Build history of the part. All positions in model axes, mm. Give positions to 0.01 mm unless a question says otherwise; leave off trailing zeros. Loops run counter-clockwise (first coordinate to the right, second up) from the corner with the lowest first, then second, coordinate; pieces in that order, holes last. Notation, with made-up numbers: M 79.25,12 L 113.25,12 A7 ccw 113.25,21 Z; hole C 46,86.25 d1. An arc over 180 degrees is marked long. Answer as a JSON object with one key per item and string values. Group by question number.
1. Drop flat-ended pins along their axis: pin 1 Ø2.5 at (x, y) = (-10.61, 259.5) entering from +Z; pin 2 Ø4.5 at (x, y) = (19.14, 230.6) entering from +Z. Give the stop position or say it passes through.
2. Slice it at B-B (z = 54.9). Give the number of separate pieces and of enclosed holes in the cut face, then the cut area to 3 significant figures.
3. Drill centre lines: line 1 along X through (y, z) = (248, 54.05); line 2 along X through (y, z) = (259, 55.2); line 3 along X through (y, z) = (231, 55.5). Where is each one in solid material? Low to high. Write a range as [from, to].
4. Slice it at C-C (x = -13). List the corners of the cut face in (y, z).
5. Slice it at A-A (x = 9). List the corners of the cut face in (y, z).
6. Mould opens along X. For faces 1 (the face through (34.622, 229.133, 54.721)), 2 (the face through (-28, 226.353, 55)), 3 (the face through (-41.107, 257, 55)) say: released by +X, released by -X, zero draft, split by the parting line, or undercut.
from build123d import *

# Parameters (mm, degrees)
SKETCH_1_R                                   = 3
SKETCH_1_R_2                                 = 4.5
EXTRUDE_1_DEPTH                              = 3
CSK_FOR_M3_HEX_SOCKET_COUNTERSUNK_HE_2_COUNT = 2
CSK_FOR_M3_HEX_SOCKET_COUNTERSUNK_HE_2_PITCH = 42.898135158
SKETCH_2_R                                   = 1.5
SKETCH_2_R_2                                 = 1.25
CUT_EXTRUDE1_DEPTH                           = 10
SKETCH4_R                                    = 1.25
CUT_EXTRUDE2_DEPTH                           = 3


with BuildPart() as part:
    # Эскиз1 → Бобышка-Вытянуть1 (new body)
    with BuildSketch(Plane.XY.offset(53.2)):
        with BuildLine():
            Line((-4.102180416, 226.353254388), (38.893407272, 226.353254388))
            Line((38.893407272, 226.353254388), (38.893407272, 286.353254388))
            Line((38.893407272, 286.353254388), (-41.106592728, 286.353254388))
            Line((-41.106592728, 286.353254388), (-41.106592728, 226.353254388))
            Line((-41.106592728, 226.353254388), (-15.28891158, 226.353254388))
            ThreePointArc((-15.28891158, 226.353254388), (-9.695545998, 229.144425829), (-4.102180416, 226.353254388))
        make_face()
        with Locations((0.393407272, 249.403254388)):
            Circle(SKETCH_1_R, mode=Mode.SUBTRACT)
        with Locations((14.393407272, 249.403254388)):
            Circle(SKETCH_1_R, mode=Mode.SUBTRACT)
        with Locations((-29.150473778, 261.95614373)):
            Circle(SKETCH_1_R_2, mode=Mode.SUBTRACT)
        with Locations((10.923063266, 261.985726175)):
            Circle(SKETCH_1_R_2, mode=Mode.SUBTRACT)
    extrude(amount=EXTRUDE_1_DEPTH)

    # Sketch3 → CSK for M3 Hex Socket Countersunk Head Screw1 (revolve, cut)
    with BuildSketch(Plane(origin=(3.643407272, 270.603254388, 56.2), x_dir=(0, -1, 0), z_dir=(1, 0, 0))):
        Polygon((0, 0), (0, 3), (1.7, 3), (1.7, 1.77), (3.47, 0), align=None)
    csk_for_m3_hex_socket_countersunk_head_s = revolve(axis=Axis((3.643407272, 270.603254388, 62.55), (0, 0, -1)), mode=Mode.SUBTRACT)

    # CSK for M3 Hex Socket Countersunk He 2: CSK for M3 Hex Socket Countersunk Head Screw1 ×2
    with Locations(*[Vector(0.36132106775864725, -0.9324414651836066, 0) * (i * CSK_FOR_M3_HEX_SOCKET_COUNTERSUNK_HE_2_PITCH) for i in range(1, CSK_FOR_M3_HEX_SOCKET_COUNTERSUNK_HE_2_COUNT)]):
        add(csk_for_m3_hex_socket_countersunk_head_s, mode=Mode.SUBTRACT)

    # Эскиз2 → Cut-Extrude1 (cut)
    with BuildSketch(Plane.XY.offset(56.2)):
        with Locations((-28.106592728, 240.603254388)):
            Circle(SKETCH_2_R)
        with Locations((-10.606592728, 259.503254388)):
            Circle(SKETCH_2_R)
        with Locations((3.643407272, 270.603254388)):
            Circle(SKETCH_2_R_2)
        with Locations((19.143407272, 230.603254388)):
            Circle(SKETCH_2_R_2)
    extrude(amount=-CUT_EXTRUDE1_DEPTH, mode=Mode.SUBTRACT)

    # Sketch4 → Cut-Extrude2 (cut)
    with BuildSketch(Plane.XY.offset(56.2)):
        with Locations((-9.606592728, 276.603254388)):
            Circle(SKETCH4_R)
        with Locations((-19.620743586, 239.653254388)):
            Circle(SKETCH4_R)
        with Locations((34.893407272, 230.353254388)):
            Circle(SKETCH4_R)
    extrude(amount=-CUT_EXTRUDE2_DEPTH, mode=Mode.SUBTRACT)


solid = part.part
Established:
{
 "1": {"pin 1": "passes through", "pin 2": "stops at z = 54.98"},
 "2": {"separate pieces": "1", "enclosed holes": "11", "area": "4,540 mm^2"},
 "3": {"line 1": "x = [-41.11, -2.26], [3.04, 11.74], [17.04, 38.89]", "line 2": "x = [-41.11, -32.54], [-25.76, -12.02], [-9.19, 7.56], [14.29, 38.89]", "line 3": "x = [-41.11, 16.4], [21.88, 33.82], [35.96, 38.89]"},
 "4": {"outline": "M 228.32,53.2 L 286.35,53.2 L 286.35,56.2 L 228.32,56.2 Z"},
 "5": {"outline": "M 226.35,53.2 L 257.92,53.2 L 257.92,56.2 L 226.35,56.2 Z; M 266.05,53.2 L 286.35,53.2 L 286.35,56.2 L 266.05,56.2 Z"},
 "6": {"face 1": "undercut", "face 2": "zero draft", "face 3": "released by -X"}
}
